from build123d import *

# Parameters (mm, degrees)
F1_DEPTH = 50.8
F3_DEPTH = 50.8


with BuildPart() as f1:
    # F0 (on Front) → F1 (new body)
    with BuildSketch(Plane.XZ):
        Polygon((0, 50.8), (0, 0), (304.8, 0), (304.8, 19.05), (127, 50.8), align=None)
    extrude(amount=-F1_DEPTH)

    # F2 (on face) → F3 (cut)
    with BuildSketch(Plane.XY.offset(50.8)):
        with BuildLine():
            add(Edge.make_bspline(
                [(0, 0), (21.1666666667, 7.1091600694), (63.5, 21.3274802081), (105.8333333333, 7.1091600694), (127, 0)],
                knots=[0, 0, 0, 0, 0.5, 1, 1, 1, 1], degree=3))
            Line((0, 0), (127, 0))
        make_face()
    extrude(amount=-F3_DEPTH, mode=Mode.SUBTRACT)


solid = f1.part
The model under review builds one solid part; all positions refer to its coordinate system, in mm. Round coordinates to 2 decimals unless told otherwise and drop trailing zeros. Loops run counter-clockwise (first coordinate to the right, second up) from the corner with the lowest first, then second, coordinate; pieces in that order, holes last. Notation, with made-up numbers: (79, 29.5) - (131, 29.5) arc R18 ccw to (131, 42.5) - close; hole circle Ø6 at (-2.5, -21.5). An arc over 180 degrees is marked (long way). Use CSV: the item, a comma, the result in double quotes.
(1) Take a section at B-B, the plane x = 254. Give the boundary of the cut face in (y, z), plus the area to 3 significant figures.
Working result:
outline,"(0, 0) - (50.8, 0) - (50.8, 28.12) - (0, 28.12) - close"
area,"1,430 mm^2"
(2) Take a section at A-A, the plane y = 18.5. Give the boundary of the cut face in (x, z), plus the area to 3 significant figures.
Working result:
outline,"(0, 0) - (304.8, 0) - (304.8, 19.05) - (127, 50.8) - (0, 50.8) - close"
area,"12,700 mm^2"
(3) Take a section at C-C, the plane x = 223.5. Give the boundary of the cut face in (y, z).
Working result:
outline,"(0, 0) - (50.8, 0) - (50.8, 33.57) - (0, 33.57) - close"
(4) For line 1 (Y direction, x = 62, z = 42.5); line 2 (Z direction, x = 235.5, y = 20) (3 decimals); line 3 (Z direction, x = 243.5, y = 37.5), list the stretches that pass through material, from the lowest coordinate up.
Working result:
line 1,"y = 14.21 to 50.8"
line 2,"z = 0 to 31.425"
line 3,"z = 0 to 30"
